Part model, mm, in its own coordinate system. Give positions to 0.01 mm unless a question says otherwise; leave off trailing zeros. Order: outer loops, then holes, each group sorted by start corner. A loop starts at its lowest first (then second) coordinate and runs counter-clockwise, first axis right, second up. Notation, with made-up numbers: M 17,-38 L 56,-38 A18 ccw 56,-20 Z; hole C 13,-29 d8. An arc over 180 degrees is marked long. Answer as a JSON object with one key per item and string values.
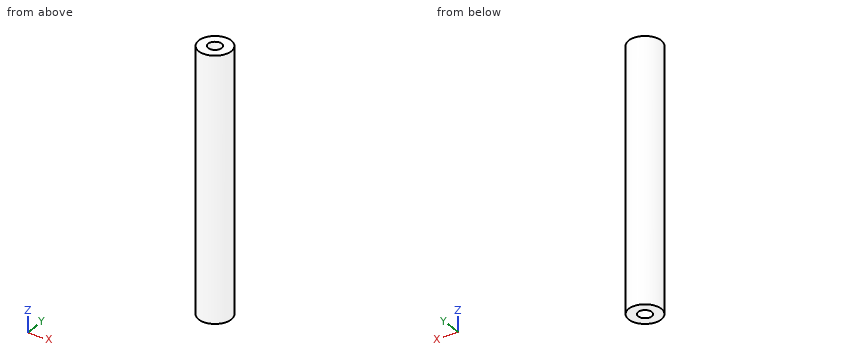
from build123d import *

# Parameters (mm, degrees)
SKETCH1_R                 = 3
BOSS_EXTRUDE1_DEPTH       = 24
M3X0_5_TAPPED_HOLE1_D     = 2.5
M3X0_5_TAPPED_HOLE1_DEPTH = 24


with BuildPart() as part:
    # Sketch1 → Boss-Extrude1 (new, symmetric)
    with BuildSketch(Plane.XY):
        Circle(SKETCH1_R)
    extrude(amount=BOSS_EXTRUDE1_DEPTH, both=True)

    # M3x0.5 Tapped Hole1
    with Locations(Plane.XY.offset(24)):
        with Locations((0, 0)):
            m3x0_5_tapped_hole1 = Hole(M3X0_5_TAPPED_HOLE1_D / 2, depth=M3X0_5_TAPPED_HOLE1_DEPTH)

    # Mirror1: M3x0.5 Tapped Hole1 across plane
    add(m3x0_5_tapped_hole1.mirror(Plane.XY), mode=Mode.SUBTRACT)


solid = part.part
1. Cut at C-C on z = -4.5. Give the cut face in (x, y), plus the area to 3 significant figures.
Worked answers:
{"outline": "C 0,0 d6; hole C 0,0 d2.5", "area": "23.4 mm^2"}
2. Probe line 1 along Y through (x, z) = (0, 11.25); line 2 along Y through (x, z) = (-0.6, -5); line 3 along Y through (x, z) = (-2.65, -17). List the from-to ranges inside material, lowest first.
Worked answers:
{"line 1": "y = -3 to -1.25, 1.25 to 3", "line 2": "y = -2.94 to -1.1, 1.1 to 2.94", "line 3": "y = -1.41 to 1.41"}
3. Cut at D-D on y = 1.9. Give the cut face in (x, z), plus the area to 3 significant figures.
Worked answers:
{"outline": "M -2.32,-24 L 2.32,-24 L 2.32,24 L -2.32,24 Z", "area": "223 mm^2"}
4. Pin check, flat tips, straight feed: P1, Ø1.5, axis at x = 2.5, z = 6, coming from the +Y side; P2, Ø2, axis at y = -2.5, z = 6.5, coming from the +X side; P3, Ø2, axis at y = 1.5, z = 8, coming from the +X side. Stop position of each tip, or through.
Worked answers:
{"P1": "stops at y = 2.44", "P2": "stops at x = 2.6", "P3": "stops at x = 2.96"}
5. Cut at A-A on y = 0. Give the cut face in (x, z), plus the area to 3 significant figures.
Worked answers:
{"outline": "M -3,-24 L -1.25,-24 L -1.25,24 L -3,24 Z; M 1.25,-24 L 3,-24 L 3,24 L 1.25,24 Z", "area": "168 mm^2"}
